Source: CAD feature listing. Evaluate the final solid. Frame: model axes, mm. A direction names the side the tool comes from. Give positions to 0.01 mm unless a question says otherwise; leave off trailing zeros. Loops run counter-clockwise (first coordinate to the right, second up) from the corner with the lowest first, then second, coordinate; pieces in that order, holes last. Notation, with made-up numbers: M -18,58.25 L 14,58.25 A16 ccw 14,80.25 Z; hole C -23.5,57.5 d8. An arc over 180 degrees is marked long. Answer in a Markdown table with one row per item.
```python
from build123d import *

# Parameters (mm, degrees)
F1_W     = 50.4830703139
F1_H     = 50.9135648608
F2_DEPTH = 25
F0_W     = 50
F0_H     = 50
F0_W_2   = 39.3322317418
F0_H_2   = 39.3322317418
F3_DEPTH = 35
F4_SIZE2 = 24.99999
F4_SIZE  = 24.99999


# Not quite as in the source:
# - a fillet or chamfer is up to 0.001 mm smaller than in the source, because OpenCascade refuses the exact size


with BuildPart() as f2:
    # F1 (on Top) → F2 (new body)
    with BuildSketch(Plane.XY):
        with Locations((25.241535157, 25.4567824304)):
            Rectangle(F1_W, F1_H)
    extrude(amount=F2_DEPTH)

    # F0 (on Top) → F3 (join)
    with BuildSketch(Plane.XY):
        with Locations((25, 25)):
            Rectangle(F0_W, F0_H)
        with Locations((24.6661158709, 24.6661158709)):
            Rectangle(F0_W_2, F0_H_2, mode=Mode.SUBTRACT)
    extrude(amount=-F3_DEPTH)

    # F4 (size 25 and 25 in the source; OpenCascade refuses exactly that, so slightly less here)
    f4_edges = [f2.edges().sort_by_distance(p)[0] for p in [
        (50.48307, 25.456782, 25),
        (0, 25.456782, 25),
    ]]
    chamfer(f4_edges, length=F4_SIZE, length2=F4_SIZE2)


solid = f2.part
```
1) Set-up query: faces 1 (the flat face through (47, 25, -35)), 2 (the flat face through (5, 24, -17)), 3 (the flat face through (25, 50, -17)), 4 (the flat face through (50, 25, -17)), 5 (the flat face through (0, 25, -17)). Return all of +Z, -Z, +X, -X, +Y, -Y with unobstructed straight access to the full face (end or side cutting, diameter ignored); none if empty.
Reply:
| item | result |
|---|---|
| face 1 | -Z, +X, -X, +Y, -Y |
| face 2 | -Z |
| face 3 | -Z, +X, -X, +Y |
| face 4 | -Z, +X, +Y, -Y |
| face 5 | +Z, -Z, -X, +Y, -Y |
2) Section A-A, the plane z = -21. Return loops of the section in (x, y).
Reply:
| item | result |
|---|---|
| outline | M 0,0 L 50,0 L 50,50 L 0,50 Z; hole M 5,5 L 44.33,5 L 44.33,44.33 L 5,44.33 Z |
3) Section C-C, the plane x = 6. Return loops of the section in (y, z), then the cut area to 3 significant figures.
Reply:
| item | result |
|---|---|
| outline | M 0,-35 L 5,-35 L 5,0 L 44.33,0 L 44.33,-35 L 50,-35 L 50,0 L 50.91,0 L 50.91,6 L 0,6 Z |
| area | 679 mm² |
4) Pull-direction query (X, two-part tool) for faces 6 (the flat face through (44.332, 24, -17)), 7 (the flat face through (38.158, 25.1, 12.325)), 8 (the flat face through (25, 0, -11)), 9 (the flat face through (24, 5, -17)); classes: released by +X, released by -X, zero draft, split by the parting line, or undercut.
Reply:
| item | result |
|---|---|
| face 6 | undercut |
| face 7 | released by +X |
| face 8 | zero draft |
| face 9 | undercut |
5) Pin query (flat end, axial travel): pin 1 Ø5 at (y, z) = (36, 18) entering from +X; pin 2 Ø4 at (x, y) = (25.5, 24.5) entering from -Z; pin 3 Ø17.5 at (x, z) = (33.5, -10.5) entering from +Y. Return the tip coordinate at first contact, or that it passes through.
Reply:
| item | result |
|---|---|
| pin 1 | stops at x = 34.98 |
| pin 2 | stops at z = 0 |
| pin 3 | stops at y = 50 |
6) Material intervals for L1, parallel to Y at x = 44, z = -18.5; L2, parallel to X at y = 38, z = 4.5, sorted ascending.
Reply:
| item | result |
|---|---|
| L1 | y = 0 to 5, 44.33 to 50 |
| L2 | x = 4.5 to 45.98 |
